Geometry: final body of the model. Coordinates: model frame, mm. Face numbers are marked on the shaded views. A direction names the side the tool comes from. Round coordinates to 2 decimals unless told otherwise and drop trailing zeros. Write each loop counter-clockwise with the first axis right and the second up, starting at its lowest first coordinate (ties: lowest second). Pieces come first, ordered by that corner, then holes. Notation, with made-up numbers: (86.5, 51.25) -> (112.5, 51.25) arc R32 ccw to (112.5, 90.25) -> close; hole circle Ø6 at (28, 72). An arc over 180 degrees is marked (long way). Use one line per item in the form item = value. Start each with the question number.
1. Reachability of the marked faces 1, 2 and 3 from +Z, -Z, +X, -X, +Y, -Y: full face, straight path, thin tool, end or side. Return the list, or none.
2. Cut plane B-B, the plane x = 191. Return the cut outline in (y, z).
3. Cut plane C-C, the plane y = 17.5. Return the cut outline in (x, z).
4. Line query: L1, parallel to Y at x = 85.5, z = -0.5; L2, parallel to Z at x = 140, y = 1. Output: solid intervals per line, ascending.
5. Cut plane A-A, the plane y = 0. Return the cut outline in (x, z), plus the area to 3 significant figures.
6. Pin query (flat end, axial travel): pin 1 Ø1.4 at (y, z) = (7, 0) entering from -X; pin 2 Ø2 at (x, z) = (154.5, 3) entering from +Y; pin 3 Ø1.2 at (y, z) = (1.5, -6.5) entering from +X; pin 4 Ø8 at (x, z) = (176.5, 0) entering from +Y. Return the tip coordinate at first contact, or that it passes through.
```python
from build123d import *

# Parameters (mm, degrees)
SKETCH1_R           = 2.5
BOSS_EXTRUDE1_DEPTH = 5
SKETCH2_R           = 7.5
BOSS_EXTRUDE2_DEPTH = 175
BOSS_EXTRUDE3_DEPTH = 5
SKETCH4_W           = 105
SKETCH4_H           = 1.8
CUT_EXTRUDE1_DEPTH  = 1.8


with BuildPart() as part:
    # Sketch1 → Boss-Extrude1 (new body)
    with BuildSketch(Plane(origin=(0, 0, 0), x_dir=(0, 0, -1), z_dir=(1, 0, 0))):
        Circle(SKETCH1_R)
    extrude(amount=BOSS_EXTRUDE1_DEPTH)

    # Sketch2 → Boss-Extrude2 (add)
    with BuildSketch(Plane(origin=(5, 0, 0), x_dir=(0, 0, -1), z_dir=(1, 0, 0))):
        Circle(SKETCH2_R)
    extrude(amount=BOSS_EXTRUDE2_DEPTH)

    # Sketch3 → Boss-Extrude3 (add, symmetric)
    with BuildSketch(Plane.XY):
        with BuildLine():
            Line((180, -25), (180, 25))
            ThreePointArc((180, 25), (205, 0), (180, -25))
        make_face()
    extrude(amount=BOSS_EXTRUDE3_DEPTH, both=True)

    # Sketch4 → Cut-Extrude1 (cut)
    with BuildSketch(Plane(origin=(0, 5.7, 0), x_dir=(1, 0, 0), z_dir=(0, 1, 0))):
        with Locations((60, 0)):
            Rectangle(SKETCH4_W, SKETCH4_H)
    cut_extrude1 = extrude(amount=CUT_EXTRUDE1_DEPTH, mode=Mode.SUBTRACT)

    # Mirror1: Cut-Extrude1 across plane
    add(cut_extrude1.mirror(Plane.ZX), mode=Mode.SUBTRACT)


solid = part.part
```
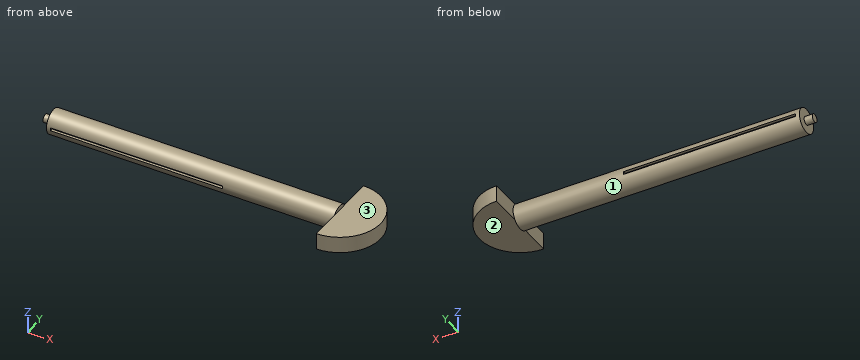
Outcome:
q1.face_1 = -X
q1.face_2 = -Z, +X, +Y, -Y
q1.face_3 = +Z, +X, +Y, -Y
q2.outline = (-22.45, -5) -> (22.45, -5) -> (22.45, 5) -> (-22.45, 5) -> close
q3.outline = (180, -5) -> (197.85, -5) -> (197.85, 5) -> (180, 5) -> close
q4.L1 = -5.7 to 5.7
q4.L2 = -7.43 to 7.43
q5.outline = (0, -2.5) -> (5, -2.5) -> (5, -7.5) -> (180, -7.5) -> (180, -5) -> (205, -5) -> (205, 5) -> (180, 5) -> (180, 7.5) -> (5, 7.5) -> (5, 2.5) -> (0, 2.5) -> close
q5.area = 2,900 mm^2
q6.pin_1 = 5
q6.pin_2 = 7.23
q6.pin_3 = 180
q6.pin_4 = 25
